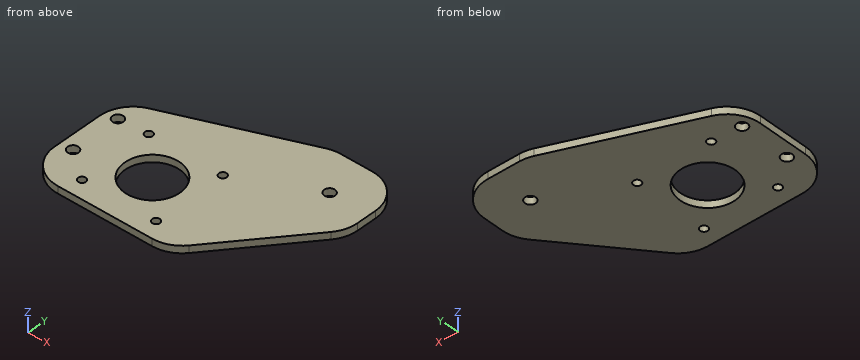
from build123d import *

# Parameters (mm, degrees)
PAD004_DEPTH         = 3
SKETCH004_R          = 2.25
SKETCH004_R_2        = 1.6
SKETCH004_R_3        = 11.5
POCKET002_DEPTH      = 0.001
POCKET002_DEPTH_BACK = 3.001
FILLET001_R          = 14


with BuildPart() as part:
    # Sketch003 → Pad004 (new body)
    with BuildSketch(Plane.XY):
        Polygon((-79.04016, -9.81434), (-79.04016, -54.156483), (-18.88891, -54.156483), (16.695431, -10.559778), (16.695431, 16.776531), (-13.233119, 16.776531), align=None)
    extrude(amount=PAD004_DEPTH)

    # Sketch004 → Pocket002 (cut, two sides)
    with BuildSketch(Plane.XY) as pocket002_sk:
        Circle(SKETCH004_R)
        with Locations((-61.528467, -15.781639)):
            Circle(SKETCH004_R_2)
        with Locations((-30.528467, -15.781639)):
            Circle(SKETCH004_R_2)
        with Locations((-61.528467, -46.781639)):
            Circle(SKETCH004_R_2)
        with Locations((-30.528467, -46.781639)):
            Circle(SKETCH004_R_2)
        with Locations((-46.028467, -31.281639)):
            Circle(SKETCH004_R_3)
        with Locations((-73.757385, -16.564894)):
            Circle(SKETCH004_R)
        with Locations((-73.757385, -37.402451)):
            Circle(SKETCH004_R)
    extrude(amount=-POCKET002_DEPTH, mode=Mode.SUBTRACT)
    extrude(pocket002_sk.sketch, amount=POCKET002_DEPTH_BACK, mode=Mode.SUBTRACT)

    # Fillet001
    fillet001_edges = [part.edges().sort_by_distance(p)[0] for p in [
        (-79.04016, -54.156483, 1.5),
        (-79.04016, -9.81434, 1.5),
        (-18.88891, -54.156483, 1.5),
        (16.695431, -10.559778, 1.5),
        (16.695431, 16.776531, 1.5),
        (-13.233119, 16.776531, 1.5),
    ]]
    fillet(fillet001_edges, radius=FILLET001_R)


with BuildPart() as part_1:
    # Body003 placement: moved
    add(part.part.moved(Location((0, 0, -16.7))))


solid = part_1.part
Could you check a few things on this model? Use its own coordinates, in mm. Round coordinates to 2 decimals unless told otherwise and drop trailing zeros. Order: outer loops, then holes, each group sorted by start corner. A loop starts at its lowest first (then second) coordinate and runs counter-clockwise, first axis right, second up.
(1) Imagine slicing it at B-B (x = -45). Write out the boundary of the cut face in (y, z).
Response values:
outline: (-54.16, -16.7) - (-42.74, -16.7) - (-42.74, -13.7) - (-54.16, -13.7) - close; (-19.83, -16.7) - (3.94, -16.7) - (3.94, -13.7) - (-19.83, -13.7) - close
(2) Imagine slicing it at A-A (y = -26.5). Write out the boundary of the cut face in (x, z), plus the area to 3 significant figures.
Response values:
outline: (-79.04, -16.7) - (-56.49, -16.7) - (-56.49, -13.7) - (-79.04, -13.7) - close; (-35.57, -16.7) - (3.68, -16.7) - (3.68, -13.7) - (-35.57, -13.7) - close
area: 185 mm2
(3) Imagine slicing it at C-C (z = -15.2). Count the separate pieces of the cut face and the enclosed holes in it, plus the area to 3 significant figures.
Response values:
separate pieces: 1
enclosed holes: 8
area: 4,540 mm2
(4) Please list where these lines run through material, in increasing order: line 1 along X through (y, z) = (-37.5, -14.4); line 2 along X through (y, z) = (-16, -13.9); line 3 along X through (y, z) = (-46, -16.05).
Response values:
line 1: x = -79.04 to -76.01, -71.51 to -55.7, -36.35 to -5.29
line 2: x = -78.66 to -75.94, -71.58 to -63.11, -59.94 to -32.11, -28.94 to 12.26
line 3: x = -77.76 to -62.92, -60.13 to -31.92, -29.13 to -12.23
(5) Imagine slicing it at D-D (y = -8.5). Write out the boundary of the cut face in (x, z), plus the area to 3 significant figures.
Response values:
outline: (-74, -16.7) - (16.39, -16.7) - (16.39, -13.7) - (-74, -13.7) - close
area: 271 mm2
